Build history of the part. All positions in model axes, mm. Round coordinates to 2 decimals unless told otherwise and drop trailing zeros. Answer as a JSON object with one key per item and string values. Group by question number.
Item 1: Flat gauge pins, fed straight in: pin 1 (10 mm diameter, centred on x = 1442, z = -36, fed in from +Y); pin 2 (10 mm diameter, centred on x = 713.359, z = -28.575, fed in from -Y); pin 3 (5 mm diameter, centred on x = 1109.5, y = 13, fed in from -Z). Where does each tip first touch, or does it go through?
Item 2: Probe line 1 (X direction, y = 7.5, z = -29) (3 decimals); line 2 (Z direction, x = 1452, y = 26); line 3 (X direction, y = 26.5, z = -6.5) (3 decimals). List the from-to ranges inside material, lowest first. Write a range as from..to.
Item 3: Two-plate mould, pull along Z, no slides. Class faces 1 (the cylindrical face through (890.178, 12.704, -28.924)), 2 (the flat face through (897, 28.575, -45)), 3 (the cylindrical face through (1781.49, 4.77, -28.05)): +Z half, -Z half, draft (parallel to the pull), parting line (faces both ways), or undercut.
from build123d import *

# Parameters (mm, degrees)
SKETCH1_W                     = 1803.4
SKETCH1_H                     = 57.15
WOOD_BLOCK_DEPTH              = 28.575
SKETCH5_R                     = 6.35
MOUTHPIECE_THROUGH_HOLE_DEPTH = 1805.531577204
SKETCH6_R                     = 3.175
DOWEL_PIN_HOLE_DEPTH          = 15.24
SKETCH8_R                     = 8.128
CUT_EXTRUDE1_DEPTH            = 10.3124
SKETCH3_OUTSIDE_W             = 420.056
SKETCH3_OUTSIDE_H             = 391.481
SKETCH3_OUTSIDE_R             = 23.8125
OUTER_DIAMETER_DEPTH          = 1805.531577305
SKETCH7_W                     = 3.175
SKETCH7_H                     = 6.35


with BuildPart() as part:
    # Sketch1 → wood block (new body)
    with BuildSketch(Plane(origin=(0, 0, 0), x_dir=(1, 0, 0), z_dir=(0, 1, 0))):
        with Locations((901.7, 28.575)):
            Rectangle(SKETCH1_W, SKETCH1_H)
    extrude(amount=WOOD_BLOCK_DEPTH)

    # Sketch2 → inner bore (revolve, cut)
    with BuildSketch(Plane.XY.offset(-28.575)):
        with BuildLine():
            Line((1771.65, 28.575), (-15.875, 28.575))
            ThreePointArc((-15.875, 28.575), (-11.225320151, 17.349679849), (0, 12.7))
            Line((0, 12.7), (1755.775, 12.7))
            ThreePointArc((1755.775, 12.7), (1767.000320151, 17.349679849), (1771.65, 28.575))
        make_face()
    revolve(axis=Axis((1771.65, 28.575, -28.575), (-1, 0, 0)), mode=Mode.SUBTRACT)

    # Sketch5 → mouthpiece through hole (cut, through all)
    with BuildSketch(Plane(origin=(0, 0, 0), x_dir=(1, 0, 0), z_dir=(0, 1, 0))):
        with Locations(Location((22.225, 28.575, 0), (0, 0, 90))):
            Circle(SKETCH5_R)
    extrude(amount=MOUTHPIECE_THROUGH_HOLE_DEPTH, mode=Mode.SUBTRACT)

    # Sketch6 → dowel pin hole (cut)
    with BuildSketch(Plane(origin=(0, 28.575, 0), x_dir=(1, 0, 0), z_dir=(0, 1, 0))):
        with Locations(Location((1787.525, 28.575, 0), (0, 0, 270))):
            Circle(SKETCH6_R)
    extrude(amount=-DOWEL_PIN_HOLE_DEPTH, mode=Mode.SUBTRACT)

    # Sketch8 → Cut-Extrude1 (cut)
    with BuildSketch(Plane.XZ):
        with Locations(Location((22.225, -28.575, 0), (0, 0, 270))):
            Circle(SKETCH8_R)
        with Locations(Location((713.359, -28.575, 0), (0, 0, 270))):
            Circle(SKETCH8_R)
    extrude(amount=-CUT_EXTRUDE1_DEPTH, mode=Mode.SUBTRACT)

    # Sketch3 outside → outer diameter (cut, through all)
    with BuildSketch(Plane(origin=(1803.4, 0, 0), x_dir=(0, 0, -1), z_dir=(1, 0, 0))):
        with Locations((28.575, 14.2875)):
            Rectangle(SKETCH3_OUTSIDE_W, SKETCH3_OUTSIDE_H)
        with Locations((28.575, 28.575)):
            Circle(SKETCH3_OUTSIDE_R, mode=Mode.SUBTRACT)
    extrude(amount=-OUTER_DIAMETER_DEPTH, mode=Mode.SUBTRACT)

    # Sketch7 → end length locator (revolve, cut)
    with BuildSketch(Plane(origin=(0, 28.575, 0), x_dir=(1, 0, 0), z_dir=(0, 1, 0))):
        with Locations((1757.3625, 7.9375)):
            Rectangle(SKETCH7_W, SKETCH7_H)
    revolve(axis=Axis((0, 28.575, -28.575), (1, 0, 0)), mode=Mode.SUBTRACT)


solid = part.part
Geometry says:
{
 "1": {"pin 1": "stops at y = 18.69", "pin 2": "stops at y = 10.31", "pin 3": "stops at z = -48.48"},
 "2": {"line 1": "x = 0..14.108, 30.342..705.242, 721.476..1755.775, 1758.95..1803.4", "line 2": "z = -52.25..-44.24, -12.91..-4.9", "line 3": "x = 0..1755.775, 1758.95..1803.4"},
 "3": {"face 1": "undercut", "face 2": "draft", "face 3": "parting line"}
}
